Check sheet for the modelled part. Datum: model origin and axes. Units: mm. A direction names the side the tool comes from. Round coordinates to 2 decimals unless told otherwise and drop trailing zeros. Write each loop counter-clockwise with the first axis right and the second up, starting at its lowest first coordinate (ties: lowest second). Pieces come first, ordered by that corner, then holes. Notation, with made-up numbers: M -20,42 L 22,42 A16 ccw 22,71 Z; hole C 34.25,31.5 d7. An arc over 180 degrees is marked long. Answer in a Markdown table with one row per item.
```python
from build123d import *

# Parameters (mm, degrees)
SKETCH1_W           = 70
SKETCH1_H           = 70
SKETCH1_R           = 2.75
BOSS_EXTRUDE1_DEPTH = 5.08
FILLET1_R           = 5


with BuildPart() as part:
    # Sketch1 → Boss-Extrude1 (new body)
    with BuildSketch(Plane(origin=(0, 0, 0), x_dir=(1, 0, 0), z_dir=(0, 1, 0))):
        with Locations((35, 35)):
            Rectangle(SKETCH1_W, SKETCH1_H)
        with Locations(Location((6, 64, 0), (0, 0, 270))):
            Circle(SKETCH1_R, mode=Mode.SUBTRACT)
        with Locations(Location((64, 64, 0), (0, 0, 270))):
            Circle(SKETCH1_R, mode=Mode.SUBTRACT)
        with Locations(Location((64, 6, 0), (0, 0, 270))):
            Circle(SKETCH1_R, mode=Mode.SUBTRACT)
        with Locations(Location((6, 6, 0), (0, 0, 270))):
            Circle(SKETCH1_R, mode=Mode.SUBTRACT)
        with BuildLine():
            Line((34, 48), (36, 48))
            ThreePointArc((36, 48), (49, 35), (36, 22))
            Line((36, 22), (34, 22))
            ThreePointArc((34, 22), (21, 35), (34, 48))
        make_face(mode=Mode.SUBTRACT)
    extrude(amount=BOSS_EXTRUDE1_DEPTH)

    # Fillet1
    fillet1_edges = [part.edges().sort_by_distance(p)[0] for p in [
        (0, 2.54, -70),
        (70, 2.54, -70),
        (70, 2.54, 0),
        (0, 2.54, 0),
    ]]
    fillet(fillet1_edges, radius=FILLET1_R)


solid = part.part
```
1. Section check A-A, the plane x = 64. Record the cut outline in (y, z).
Found:
| item | result |
|---|---|
| outline | M 0,-70 L 5.08,-70 L 5.08,-66.75 L 0,-66.75 Z; M 0,-61.25 L 5.08,-61.25 L 5.08,-8.75 L 0,-8.75 Z; M 0,-3.25 L 5.08,-3.25 L 5.08,0 L 0,0 Z |
2. Draft check along Z on faces 1 (the face through (1, 3, -68)), 2 (the face through (35, 5.08, -51)), 3 (the face through (1, 3, -2)), 4 (the face through (35, 3, -48)). Enter one of: +Z half, -Z half, draft (parallel to the pull), parting line (faces both ways), or undercut.
Found:
| item | result |
|---|---|
| face 1 | -Z half |
| face 2 | draft |
| face 3 | +Z half |
| face 4 | undercut |
3. Access from +Z, -Z, +X, -X, +Y, -Y to the whole of each face (thin tool, end or side, straight path). Record for faces 5 (the face through (21, 3, -35)), 6 (the face through (68, 3, -69)).
Found:
| item | result |
|---|---|
| face 5 | +Y, -Y |
| face 6 | -Z, +X, +Y, -Y |
4. Section check D-D, the plane z = -35. Record the cut outline in (x, y).
Found:
| item | result |
|---|---|
| outline | M 0,0 L 21,0 L 21,5.08 L 0,5.08 Z; M 49,0 L 70,0 L 70,5.08 L 49,5.08 Z |
5. Section check B-B, the plane y = 2.2. Record the cut outline in (x, z), and give its area (3 significant figures).
Found:
| item | result |
|---|---|
| outline | M 0,-65 A5 ccw 5,-70 L 65,-70 A5 ccw 70,-65 L 70,-5 A5 ccw 65,0 L 5,0 A5 ccw 0,-5 Z; hole C 6,-64 d5.5; hole C 6,-6 d5.5; hole M 34,-48 L 36,-48 A13 ccw 36,-22 L 34,-22 A13 ccw Z; hole C 64,-64 d5.5; hole C 64,-6 d5.5 |
| area | 4,200 mm2 |
6. Section check C-C, the plane z = -6. Record the cut outline in (x, y).
Found:
| item | result |
|---|---|
| outline | M 0,0 L 3.25,0 L 3.25,5.08 L 0,5.08 Z; M 8.75,0 L 61.25,0 L 61.25,5.08 L 8.75,5.08 Z; M 66.75,0 L 70,0 L 70,5.08 L 66.75,5.08 Z |
7. Scan lines: L1, parallel to X at y = 1.15, z = -64; L2, parallel to Z at x = 34, y = 3.8; L3, parallel to Z at x = 8, y = 4.6. Record each from-to range of solid material in increasing order.
Found:
| item | result |
|---|---|
| L1 | x = 0 to 3.25, 8.75 to 61.25, 66.75 to 70 |
| L2 | z = -70 to -48, -22 to 0 |
| L3 | z = -70 to -65.89, -62.11 to -7.89, -4.11 to 0 |
